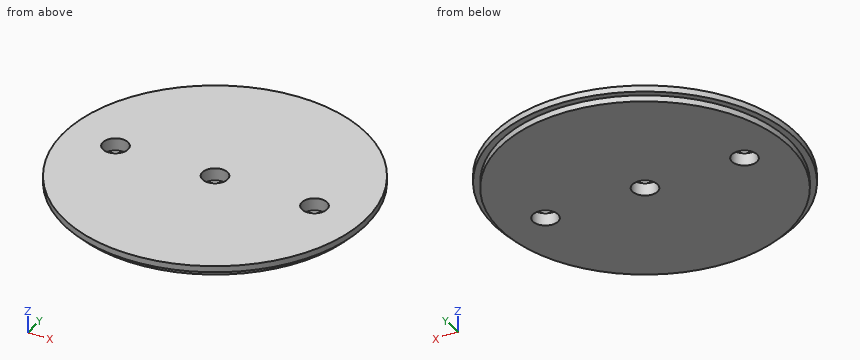
from build123d import *

# Parameters (mm, degrees)
SKETCH1_R           = 38.1
BOSS_EXTRUDE1_DEPTH = 3.175
SKETCH2_R           = 38.1
SKETCH2_R_2         = 36.5125
CUT_EXTRUDE1_DEPTH  = 1.5875
SKETCH3_R           = 3.175
CUT_EXTRUDE2_DEPTH  = 54.975


with BuildPart() as part:
    # Sketch1 → Boss-Extrude1 (new body)
    with BuildSketch(Plane.XY):
        Circle(SKETCH1_R)
    extrude(amount=BOSS_EXTRUDE1_DEPTH)

    # Sketch2 → Cut-Extrude1 (cut)
    with BuildSketch(Plane(origin=(0, 0, 0), x_dir=(-1, 0, 0), z_dir=(0, 0, -1))):
        Circle(SKETCH2_R)
        Circle(SKETCH2_R_2, mode=Mode.SUBTRACT)
    extrude(amount=-CUT_EXTRUDE1_DEPTH, mode=Mode.SUBTRACT)

    # Sketch3 → Cut-Extrude2 (cut, through all)
    with BuildSketch(Plane.XY.offset(3.175)):
        Circle(SKETCH3_R)
        with Locations((25.4, 0)):
            Circle(SKETCH3_R)
        with Locations((-25.4, 0)):
            Circle(SKETCH3_R)
    extrude(amount=-CUT_EXTRUDE2_DEPTH, mode=Mode.SUBTRACT)


solid = part.part
Design review of the part built by this model. Coordinates are the model's own, in mm. Round coordinates to 2 decimals unless told otherwise and drop trailing zeros. Loops run counter-clockwise (first coordinate to the right, second up) from the corner with the lowest first, then second, coordinate; pieces in that order, holes last. Notation, with made-up numbers: M 33.5,31.5 L 73.5,31.5 A30 cw 73.5,70.5 Z; hole C 55.5,-28.75 d2. An arc over 180 degrees is marked long. Answer as a JSON object with one key per item and string values.
Item 1: We need section D-D on y = -19.5. Give the boundary of the cut face in (x, z) (1 decimal), and give its area (3 significant figures).
Answer sheet:
{"outline": "M -32.7,1.6 L -30.9,1.6 L -30.9,0 L 30.9,0 L 30.9,1.6 L 32.7,1.6 L 32.7,3.2 L -32.7,3.2 Z", "area": "202 mm^2"}
Item 2: We need section C-C on z = 2.45. Give the boundary of the cut face in (x, y) (3 decimals).
Answer sheet:
{"outline": "C 0,0 d76.2; hole C -25.4,0 d6.35; hole C 0,0 d6.35; hole C 25.4,0 d6.35"}
Item 3: We need section B-B on y = 0. Give the boundary of the cut face in (x, z) (1 decimal).
Answer sheet:
{"outline": "M -38.1,1.6 L -36.5,1.6 L -36.5,0 L -28.6,0 L -28.6,3.2 L -38.1,3.2 Z; M -22.2,0 L -3.2,0 L -3.2,3.2 L -22.2,3.2 Z; M 3.2,0 L 22.2,0 L 22.2,3.2 L 3.2,3.2 Z; M 28.6,0 L 36.5,0 L 36.5,1.6 L 38.1,1.6 L 38.1,3.2 L 28.6,3.2 Z"}
Item 4: Wall thickness on L1, parallel to Y at x = 0, z = 0.9 (1 decimal); L2, parallel to X at y = 2, z = 2.15; L3, parallel to Y at x = 0, z = 2.45 (3 decimals): over which ranges is each line inside the solid? List them lowest first. Write a range as from..to.
Answer sheet:
{"L1": "y = -36.5..-3.2, 3.2..36.5", "L2": "x = -38.05..-27.87, -22.93..-2.47, 2.47..22.93, 27.87..38.05", "L3": "y = -38.1..-3.175, 3.175..38.1"}
Item 5: Clearance check with flat-ended pins moving along their axes: P1, Ø1.5, axis at x = 19.5, z = 1.5, coming from the -Y side; P2, Ø1.5, axis at x = -3.5, z = 2, coming from the -Y side; P3, Ø1, axis at y = -12.5, z = 1.5, coming from the +X side. State where each tip first meets the part, or that it passes through.
Answer sheet:
{"P1": "stops at y = -33.16", "P2": "stops at y = -38", "P3": "stops at x = 36.16"}
Item 6: We need section A-A on x = 0. Give the boundary of the cut face in (y, z) (1 decimal).
Answer sheet:
{"outline": "M -38.1,1.6 L -36.5,1.6 L -36.5,0 L -3.2,0 L -3.2,3.2 L -38.1,3.2 Z; M 3.2,0 L 36.5,0 L 36.5,1.6 L 38.1,1.6 L 38.1,3.2 L 3.2,3.2 Z"}
